Autodesk Inventor part; units mm, degrees
ref_plane "XZ Plane" through (0, 0, 0) normal (0, 1, 0) x (-1, 0, 0)
ref_plane "XY Plane" through (0, 0, 0) normal (0, 0, 1) x (1, 0, 0)
ref_plane "Work Plane1" through (0, 0, -3.25) normal (0, 0, -1) x (-1, 0, 0)
sketch "Sketch1" plane through (0, 0, 0) normal (0, 0, 1) x (1, 0, 0)
  line L0 (-27.5, 6.775) -> (27.5, 6.775)
  line L1 (27.5, 6.775) -> (27.5, -5.925)
  line L2 (27.5, -5.925) -> (-27.5, -5.925)
  line L3 (-27.5, -5.925) -> (-27.5, 6.775)
  point P0 (0, 0)
  dimension "d0" = 6.775
  dimension "d1" = 5.925
  dimension "d2" = 27.5
  dimension "d3" = 27.5
extrude "Extrusion1" add sketch "Sketch1" along normal blind 10
ref_plane "Work Plane1" through (0, 0, -3.25) normal (0, 0, -1) x (-1, 0, 0)
sketch "Sketch2" plane through (0, 0, -3.25) normal (0, 0, -1) x (-1, 0, 0)
  line L0 (27.5, 6.775) -> (-27.5, 6.775)
  line L1 (-27.5, -5.925) -> (27.5, -5.925)
  line L2 (0, 6.775) -> (-8.1, 6.775)
  line L3 (-27.5, 6.775) -> (27.5, 6.775)
  line L4 (-8.1, 6.775) -> (-8.1, 2.825)
  line L5 (-8.1, 2.825) -> (-6.25, 2.825)
  line L6 (-6.25, 2.825) -> (-6.25, -2.825)
  line L7 (-6.25, -2.825) -> (-8.1, -2.825)
  line L8 (-8.1, -2.825) -> (-8.1, -5.925)
  line L9 (27.5, -5.925) -> (-27.5, -5.925)
  line L10 (-8.1, -5.925) -> (0, -5.925)
  line L11 (0, -5.925) -> (0, 6.775)
  line L12 (0, -8.465) -> (0, 9.315)
  point P0 (0, 0)
  dimension "d7" = 8.1
  dimension "d8" = 6.25
  dimension "d9" = 3.95
  dimension "d10" = 3.1
revolve "Revolution1" cut sketch "Sketch2" angle 180 about axis through (0, 0, -3.25) along (0, -1, 0)
sketch "Sketch3" plane through (0, 0, 10) normal (0, 0, 1) x (1, 0, 0)
  line L0 (0, 0) -> (43.2339, 0) construction
  line L1 (0, 0) -> (-39.8542, 0) construction
  point P0 (-12.5, 0)
  point P1 (12.5, 0)
  dimension "d12" = 12.5
  dimension "d13" = 12.5
hole "Hole1" at (-12.5, 0, 10) at (12.5, 0, 10) direction (0, 0, -1) diameter 3.5 end through all counterbore diameter 6.5 counterbore depth 3
sketch "Sketch5" plane through (-27.5, 6.775, 10) normal (0, 1, 0) x (1, 0, 0)
  arc A0 (22.1615, 10) -> (32.8385, 10) centre (27.5, 13.25) ccw
  line L0 (27.5, 13.25) -> (61.0026, 13.25) construction
  line L1 (55, 10) -> (55, 0)
  circle A1 centre (49, 13.25) radius 5.5
  point P0 (27.5, 10)
  dimension "d26" = 6
  dimension "d27" = 11
extrude "Extrusion3" cut sketch "Sketch5" against normal through all
sketch "Sketch6" plane through (-12.5, 0, 7) normal (0, 0, 1) x (1, 0, 0)
  circle A0 centre (0, 0) radius 1.75
  circle A1 centre (25, 0) radius 1.75
  point P0 (12.5, 0)
extrude "Extrusion4" add sketch "Sketch6" against normal blind 0.4
fillet "Fillet2" radius 1 4 edges at (-27.5, 6.775, 5) (-27.5, -5.925, 5) (27.5, 6.775, 5) (27.5, -5.925, 5)
properties part number "Retainer" material "PC/ABS Plastic"
CAD build for the part. Positions are in the model's coordinates, mm. A direction names the side the tool comes from. Round coordinates to 2 decimals unless told otherwise and drop trailing zeros. Write each loop counter-clockwise with the first axis right and the second up, starting at its lowest first coordinate (ties: lowest second). Pieces come first, ordered by that corner, then holes.
(1) Slice it at D-D, the plane y = 0. Write the cut outline in (x, z), and give its area (3 significant figures).
(2) Probe line 1 along X through (y, z) = (0, 4); line 2 along Y through (x, z) = (12.5, 8.05) (3 decimals); line 3 along Y through (x, z) = (12.5, 2.5) (3 decimals). List the from-to ranges inside material, lowest first.
(3) Drop flat-ended pins along their axis: P1, Ø7, axis at x = -11.5, y = -0.5, coming from the +Z side; P2, Ø3, axis at x = 12.5, y = 0, coming from the -Z side; P3, Ø2.5, axis at x = -1.5, z = 2, coming from the +Y side (3 decimals); P4, Ø4, axis at x = -2.5, z = 1.5, coming from the -Y side (3 decimals). Give the stop position or say it passes through.
(4) 3-axis set-ups, long thin cutter, end or side, ignore diameter. For faces 1 (the face through (0.13, -4.4, 4.85)), 2 (the face through (-13, 0, 7)), 3 (the face through (0.13, 4.77, 4.85)), 4 (the face through (-13, 0, 6.6)): which of +Z, -Z, +X, -X, +Y, -Y reach the whole face in a straight line?
(5) Slice it at C-C, the plane z = 8.25. Write the cut outline in (x, y) (3 decimals), and give its area (3 significant figures).
(6) Slice it at B-B, the plane x = -12.5. Write the cut outline in (y, z) (3 decimals), and give its area (3 significant figures).
(7) Slice it at A-A, the plane z = 1.75. Write the cut outline in (x, y) (3 decimals).
From the geometry:
1. outline: (-27.5, 0) - (-14.25, 0) - (-14.25, 6.6) - (-10.75, 6.6) - (-10.75, 0) - (-5.34, 0) arc R6.25 cw to (5.34, 0) - (10.75, 0) - (10.75, 6.6) - (14.25, 6.6) - (14.25, 0) - (17.06, 0) arc R5.5 cw to (25.94, 0) - (27.5, 0) - (27.5, 10) - (15.75, 10) - (15.75, 7) - (9.25, 7) - (9.25, 10) - (-9.25, 10) - (-9.25, 7) - (-15.75, 7) - (-15.75, 10) - (-27.5, 10) - close
1. area: 428 mm2
2. line 1: x = -27.5 to -14.25, -10.75 to 10.75, 14.25 to 27.5
2. line 2: y = -5.925 to -3.25, 3.25 to 6.775
2. line 3: y = -5.925 to -1.75, 1.75 to 6.775
3. P1: stops at z = 10
3. P2: stops at z = 6.6
3. P3: stops at y = 2.825
3. P4: stops at y = -2.825
4. face 1: -Z, -Y
4. face 2: +Z
4. face 3: -Z, +Y
4. face 4: -Z
5. outline: (-27.5, -4.925) arc R1 ccw to (-26.5, -5.925) - (26.5, -5.925) arc R1 ccw to (27.5, -4.925) - (27.5, 5.775) arc R1 ccw to (26.5, 6.775) - (-26.5, 6.775) arc R1 ccw to (-27.5, 5.775) - close; hole circle Ø6.5 at (-12.5, 0); hole circle Ø6.5 at (12.5, 0)
5. area: 631 mm2
6. outline: (-5.925, 0) - (-1.75, 0) - (-1.75, 6.6) - (1.75, 6.6) - (1.75, 0) - (6.775, 0) - (6.775, 10) - (3.25, 10) - (3.25, 7) - (-3.25, 7) - (-3.25, 10) - (-5.925, 10) - close
6. area: 84.4 mm2
7. outline: (-27.5, -4.925) arc R1 ccw to (-26.5, -5.925) - (-6.373, -5.925) - (-6.373, -2.825) - (-3.75, -2.825) - (-3.75, 2.825) - (-6.373, 2.825) - (-6.373, 6.775) - (-26.5, 6.775) arc R1 ccw to (-27.5, 5.775) - close; (3.75, -2.825) - (6.373, -2.825) - (6.373, -5.925) - (19.209, -5.925) - (19.209, 6.775) - (6.373, 6.775) - (6.373, 2.825) - (3.75, 2.825) - close; (23.791, -5.925) - (26.5, -5.925) arc R1 ccw to (27.5, -4.925) - (27.5, 5.775) arc R1 ccw to (26.5, 6.775) - (23.791, 6.775) - close; hole circle Ø3.5 at (-12.5, 0); hole circle Ø3.5 at (12.5, 0)
